Check sheet for the modelled part. Datum: model origin and axes. Units: mm. Give positions to 0.01 mm unless a question says otherwise; leave off trailing zeros. Write each loop counter-clockwise with the first axis right and the second up, starting at its lowest first coordinate (ties: lowest second). Pieces come first, ordered by that corner, then holes. Notation, with made-up numbers: M -12,-11 L 11,-11 A22 cw 11,0 Z; hole C 57.5,7 d7. An arc over 180 degrees is marked long. Write item = value, one per line. Start each with the question number.
1) Sectioned sample at B-B, the plane x = 17. Record the cut outline in (y, z), then the cut area to 3 significant figures.
2) Sectioned sample at D-D, the plane z = 0.85. Record the cut outline in (x, y).
3) Gauge pin test, flat ends, axial feed: pin 1 (1.4 mm diameter, centred on x = 20, z = 1.5, fed in from -Y); pin 2 (1 mm diameter, centred on y = 30.5, z = 2, fed in from +X); pin 3 (0.9 mm diameter, centred on y = 13, z = 1.5, fed in from -X). Record the tip position at first contact, or that the pin passes through.
4) Sectioned sample at C-C, the plane x = 41.5. Record the cut outline in (y, z).
5) Sectioned sample at A-A, the plane y = 56. Record the cut outline in (x, z).
6) Scan lines: L1, parallel to Y at x = 20, z = 4.25; L2, parallel to X at y = 46, z = 2.9; L3, parallel to X at y = 36.5, z = 3.25. Record each from-to range of solid material in increasing order.
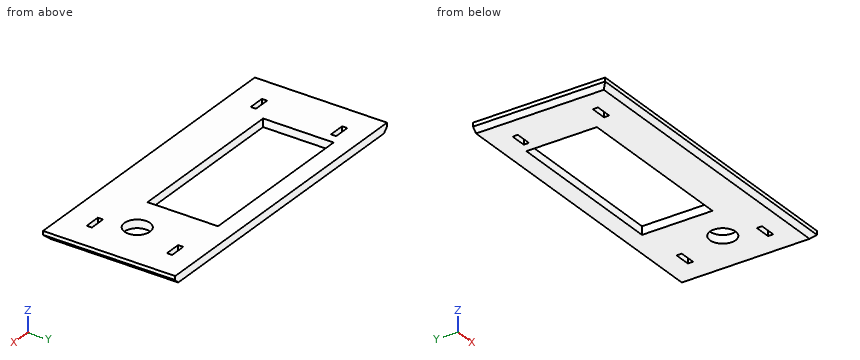
from build123d import *

# Parameters (mm, degrees)
F0_W     = 177.8
F0_H     = 76.2
F0_W_2   = 97.028
F0_H_2   = 40.64
F1_DEPTH = 4.7244
F2_R     = 7.4041
F3_DEPTH = 25.4
F4_SIZE  = 2.54
F5_W     = 9.382727
F5_H     = 2.9972
F6_DEPTH = 25.4


with BuildPart() as f1:
    # F0 (on Top) → F1 (new body)
    with BuildSketch(Plane.XY):
        with Locations((88.9, 35.43033)):
            Rectangle(F0_W, F0_H)
        with Locations((78.5368, 43.05033)):
            Rectangle(F0_W_2, F0_H_2, mode=Mode.SUBTRACT)
    extrude(amount=F1_DEPTH)

    # F2 (on face) → F3 (cut)
    with BuildSketch(Plane.XY.offset(4.7244)):
        with Locations((149.5933, 32.281343)):
            Circle(F2_R)
    extrude(amount=-F3_DEPTH, mode=Mode.SUBTRACT)

    # F4
    f4_edges = [f1.edges().sort_by_distance(p)[0] for p in [
        (0, 35.43033, 0),
        (88.9, -2.66967, 0),
        (177.8, 35.43033, 0),
    ]]
    chamfer(f4_edges, length=F4_SIZE)

    # F5 (on face) → F6 (cut)
    with BuildSketch(Plane(origin=(0, 0, 0), x_dir=(1, 0, 0), z_dir=(0, 0, -1))):
        with Locations((19.575764, -13.15453)):
            Rectangle(F5_W, F5_H)
        with Locations((19.575764, -59.40793)):
            Rectangle(F5_W, F5_H)
        with Locations((157.269163, -13.15453)):
            Rectangle(F5_W, F5_H)
        with Locations((157.269163, -59.40793)):
            Rectangle(F5_W, F5_H)
    extrude(amount=-F6_DEPTH, mode=Mode.SUBTRACT)


solid = f1.part
Data:
q1.outline = M -2.67,2.54 L -0.13,0 L 11.66,0 L 11.66,4.72 L -2.67,4.72 Z; M 14.65,0 L 57.91,0 L 57.91,4.72 L 14.65,4.72 Z; M 60.91,0 L 73.53,0 L 73.53,4.72 L 60.91,4.72 Z
q1.area = 328 mm2
q2.outline = M 1.69,-0.98 L 176.11,-0.98 L 176.11,73.53 L 1.69,73.53 Z; hole M 14.88,11.66 L 24.27,11.66 L 24.27,14.65 L 14.88,14.65 Z; hole M 14.88,57.91 L 24.27,57.91 L 24.27,60.91 L 14.88,60.91 Z; hole M 30.02,22.73 L 127.05,22.73 L 127.05,63.37 L 30.02,63.37 Z; hole C 149.59,32.28 d14.81; hole M 152.58,11.66 L 161.96,11.66 L 161.96,14.65 L 152.58,14.65 Z; hole M 152.58,57.91 L 161.96,57.91 L 161.96,60.91 L 152.58,60.91 Z
q3.pin_1 = -2.33
q3.pin_2 = 177.76
q3.pin_3 = 0.59
q4.outline = M -2.67,2.54 L -0.13,0 L 22.73,0 L 22.73,4.72 L -2.67,4.72 Z; M 63.37,0 L 73.53,0 L 73.53,4.72 L 63.37,4.72 Z
q5.outline = M 0,2.54 L 2.54,0 L 30.02,0 L 30.02,4.72 L 0,4.72 Z; M 127.05,0 L 175.26,0 L 177.8,2.54 L 177.8,4.72 L 127.05,4.72 Z
q6.L1 = -2.67 to 11.66, 14.65 to 57.91, 60.91 to 73.53
q6.L2 = 0 to 30.02, 127.05 to 177.8
q6.L3 = 0 to 30.02, 127.05 to 143.51, 155.68 to 177.8
